Model file for the job. Use its own axes, mm. A direction names the side the tool comes from. Coordinates: 2 decimals unless noted, no trailing zeros. Write each loop counter-clockwise with the first axis right and the second up, starting at its lowest first coordinate (ties: lowest second). Pieces come first, ordered by that corner, then holes. Notation, with made-up numbers: M 60,66.25 L 111,66.25 A27 ccw 111,100.25 Z; hole C 71,42.25 d8. An arc over 180 degrees is marked long. Put each result on its own line as item: value. Start each with the question number.
Q1. Cut at D-D (x = -45). Write the cut outline in (y, z).
Q2. Which spindle directions (+Z, -Z, +X, -X, +Y, -Y) get a long thin tool onto all of the face, cutting with end or side? Do faces 4 (the flat face through (-36, 16, -29.656)), 5 (the flat face through (-9, 6, -11.281)), 6 (the flat face through (-60.335, 17, -11)). Say none if no direction does.
Q3. Pull direction X, two halves, no side cores. Call faces 1 (the cylindrical face through (-28.425, -1.479, -17.461)), 2 (the flat face through (-9, 7.853, -19)), 3 (the flat face through (-7.335, 16, -11)): pulls with the +X half, pulls with the -X half, needs draft (parallel to the pull), parting line crosses it, or undercut.
Q4. Cut at B-B (x = -37.5). Write the cut outline in (y, z).
Q5. Drop flat-ended pins along their axis: pin 1 (4 mm diameter, centred on x = -57.5, z = -1.5, fed in from +Y); pin 2 (3 mm diameter, centred on x = -44.23, z = -5.59, fed in from -Y). Give the stop position or say it passes through.
Q6. Drill centre lines: line 1 along X through (y, z) = (10, 0.5); line 2 along Z through (x, y) = (-48, 22); line 3 along Y through (x, z) = (-11.5, 0). Where is each one in solid material? Low to high.
Q7. Cut at A-A (y = 31). Write the cut outline in (x, z).
Q8. Cut at C-C (z = -23). Write the cut outline in (x, y), then the cut area to 3 significant figures.
```python
from build123d import *

# Parameters (mm, degrees)
ESBO_O1_W                = 50
ESBO_O1_H                = 30
RESSALTO_EXTRUS_O1_DEPTH = 35
CASCA1_T                 = 3
ESBO_O3_W                = 15
ESBO_O3_H                = 4
CORTE_EXTRUS_O2_DEPTH    = 35
ESBO_O4_R                = 2
CORTE_EXTRUS_O3_DEPTH    = 79.203795706


with BuildPart() as part:
    # Esboço1 → Ressalto-extrusão1 (new body)
    with BuildSketch(Plane(origin=(0, 0, 0), x_dir=(1, 0, 0), z_dir=(0, 1, 0))):
        with Locations((-35.335240137, 11.656045246)):
            Rectangle(ESBO_O1_W, ESBO_O1_H)
    extrude(amount=RESSALTO_EXTRUS_O1_DEPTH)

    # Casca1
    casca1_openings = [part.faces().sort_by_distance(p)[0] for p in [
        (-35.335240137, 35, -11.656045246),
    ]]
    offset(amount=CASCA1_T, openings=casca1_openings, kind=Kind.INTERSECTION)

    # Esboço3 → Corte-extrusão2 (cut)
    with BuildSketch(Plane(origin=(-7.335240137, 0, 0), x_dir=(0, 0, -1), z_dir=(1, 0, 0))):
        with Locations((18.781461493, 5.852803371)):
            Rectangle(ESBO_O3_W, ESBO_O3_H)
    extrude(amount=-CORTE_EXTRUS_O2_DEPTH, mode=Mode.SUBTRACT)

    # Esboço4 → Corte-extrusão3 (cut, through all)
    with BuildSketch(Plane(origin=(0, 0, 0), x_dir=(1, 0, 0), z_dir=(0, 1, 0))):
        with Locations(Location((-44.228238168, 17.721247166, 0), (0, 0, 270))):
            Circle(ESBO_O4_R)
        with Locations(Location((-44.228238168, 5.590843326, 0), (0, 0, 90))):
            Circle(ESBO_O4_R)
        with Locations(Location((-26.442242107, 5.590843326, 0), (0, 0, 270))):
            Circle(ESBO_O4_R)
        with Locations(Location((-26.442242107, 17.721247166, 0), (0, 0, 90))):
            Circle(ESBO_O4_R)
    extrude(amount=-CORTE_EXTRUS_O3_DEPTH, mode=Mode.SUBTRACT)


solid = part.part
```
Computed values:
1. outline: M -3,-29.66 L 35,-29.66 L 35,-26.66 L 0,-26.66 L 0,-19.57 L -3,-19.57 Z; M -3,-15.88 L 0,-15.88 L 0,-7.44 L -3,-7.44 Z; M -3,-3.75 L 0,-3.75 L 0,3.34 L 35,3.34 L 35,6.34 L -3,6.34 Z
2. face 4: -Z, +X, -X, +Y, -Y
2. face 5: +X
2. face 6: +Y
3. face 1: undercut
3. face 2: needs draft
3. face 3: pulls with the +X half
4. outline: M -3,-29.66 L 35,-29.66 L 35,-26.66 L 0,-26.66 L 0,3.34 L 35,3.34 L 35,6.34 L -3,6.34 Z
5. pin 1: y = 0
5. pin 2: through
6. line 1: -63.34 to -60.34, -10.34 to -7.34
6. line 2: -29.66 to -26.66, 3.34 to 6.34
6. line 3: -3 to 0
7. outline: M -63.34,-29.66 L -7.34,-29.66 L -7.34,6.34 L -63.34,6.34 Z; hole M -60.34,-26.66 L -10.34,-26.66 L -10.34,3.34 L -60.34,3.34 Z
8. outline: M -63.34,-3 L -7.34,-3 L -7.34,3.85 L -10.34,3.85 L -10.34,0 L -60.34,0 L -60.34,35 L -63.34,35 Z; M -10.34,7.85 L -7.34,7.85 L -7.34,35 L -10.34,35 Z
8. area: 366 mm2
